```python
from build123d import *

# Parameters (mm, degrees)
SKETCH1_R                                  = 3
BOSS_EXTRUDE1_DEPTH                        = 275
SKETCH3_W                                  = 0.8
SKETCH3_H                                  = 0.5
CUT_EXTRUDE2_DEPTH                         = 276.032725326
CUT_EXTRUDE2_DEPTH_BACK                    = 276.032725326
SKETCH4_W                                  = 3.470061058
SKETCH4_H                                  = 7
SKETCH4_W_2                                = 2.92528695
CHAMFER1_SIZE                              = 0.3
RETAINING_GROOVES_D5P7_1_START             = 7.05
SKETCH5_R                                  = 2.85
SKETCH5_R_2                                = 2.49
RETAINING_GROOVES_D5P7_1_DEPTH             = 0.8
RETAINING_GROOVES_D5P7_2_START             = 13
SKETCH6_R                                  = 2.85
SKETCH6_R_2                                = 2.49
RETAINING_GROOVES_D5P7_2_DEPTH             = 0.8
RETAINING_GROOVES_D5P7_3_START             = 260.25
SKETCH7_R                                  = 2.85
SKETCH7_R_2                                = 2.49
RETAINING_GROOVES_D5P7_3_DEPTH             = 0.8
RETAINING_GROOVES_D5P7_4_START             = 266.2
SKETCH8_R                                  = 2.85
SKETCH8_R_2                                = 2.49
RETAINING_GROOVES_D5P7_4_DEPTH             = 0.8
TWO_HUB_CROSS_PIN_D2_DEPTH                 = 276.032725326
TWO_HUB_CROSS_PIN_D2_DEPTH_BACK            = 276.032725326
SKETCH9_R                                  = 1
SKETCH10_R                                 = 3.1
REVB_LOWER_SHAFT_NOSE_CLEARANCE_2MM_DEPTH  = 2
REVB_OLDHAM_D2_DRIVE_PIN_CLOCKED_HOLE_OU_W = 1
REVB_OLDHAM_D2_DRIVE_PIN_CLOCKED_HOLE_OU_H = 6.000106441


# Read off the part's stored shape, not the designer's step: RevB_Oldham_D2_Drive_Pin_Clocked_Hole
with BuildPart() as part:
    # Sketch1 → Boss-Extrude1 (new body)
    with BuildSketch(Plane.XY):
        Circle(SKETCH1_R)
    extrude(amount=BOSS_EXTRUDE1_DEPTH)

    # Sketch3 → Cut-Revolve1 (revolve, cut)
    with BuildSketch(Plane(origin=(0, 0, 0), x_dir=(0, 0, -1), z_dir=(1, 0, 0)), mode=Mode.PRIVATE) as cut_revolve1_sk:
        with Locations((-266.6, 2.75)):
            Rectangle(SKETCH3_W, SKETCH3_H)
        with Locations((-260.65, 2.75)):
            Rectangle(SKETCH3_W, SKETCH3_H)
        with Locations((-13.4, 2.75)):
            Rectangle(SKETCH3_W, SKETCH3_H)
        with Locations((-7.45, 2.75)):
            Rectangle(SKETCH3_W, SKETCH3_H)
    revolve(cut_revolve1_sk.sketch.rotate(Axis((0, 0, 263.365004794), (0, 0, -1)), 90), axis=Axis((0, 0, 263.365004794), (0, 0, -1)), mode=Mode.SUBTRACT)

    # Sketch4 → Cut-Extrude2 (cut, two sides: drawn at the far end of the back side and taken through both)
    with BuildSketch(Plane(origin=(0, 0, 0), x_dir=(1, 0, 0), z_dir=(0, 1, 0)).offset(-CUT_EXTRUDE2_DEPTH_BACK)):
        with Locations((4.235030529, -3.5)):
            Rectangle(SKETCH4_W, SKETCH4_H)
        with Locations((-3.962643475, -3.5)):
            Rectangle(SKETCH4_W_2, SKETCH4_H)
    extrude(amount=CUT_EXTRUDE2_DEPTH + CUT_EXTRUDE2_DEPTH_BACK, mode=Mode.SUBTRACT)

    # Chamfer1
    chamfer1_edges = [part.edges().sort_by_distance(p)[0] for p in [
        (0, 3, 0),
        (0, -3, 0),
    ]]
    chamfer(chamfer1_edges, length=CHAMFER1_SIZE)

    # Sketch5 → Retaining_Grooves_D5p7_1 (add)
    with BuildSketch(Plane.XY.offset(RETAINING_GROOVES_D5P7_1_START)):
        Circle(SKETCH5_R)
        Circle(SKETCH5_R_2, mode=Mode.SUBTRACT)
    extrude(amount=RETAINING_GROOVES_D5P7_1_DEPTH)

    # Sketch6 → Retaining_Grooves_D5p7_2 (add)
    with BuildSketch(Plane.XY.offset(RETAINING_GROOVES_D5P7_2_START)):
        Circle(SKETCH6_R)
        Circle(SKETCH6_R_2, mode=Mode.SUBTRACT)
    extrude(amount=RETAINING_GROOVES_D5P7_2_DEPTH)

    # Sketch7 → Retaining_Grooves_D5p7_3 (add)
    with BuildSketch(Plane.XY.offset(RETAINING_GROOVES_D5P7_3_START)):
        Circle(SKETCH7_R)
        Circle(SKETCH7_R_2, mode=Mode.SUBTRACT)
    extrude(amount=RETAINING_GROOVES_D5P7_3_DEPTH)

    # Sketch8 → Retaining_Grooves_D5p7_4 (add)
    with BuildSketch(Plane.XY.offset(RETAINING_GROOVES_D5P7_4_START)):
        Circle(SKETCH8_R)
        Circle(SKETCH8_R_2, mode=Mode.SUBTRACT)
    extrude(amount=RETAINING_GROOVES_D5P7_4_DEPTH)

    # Sketch9 → Two_Hub_Cross_Pin_D2 (cut, two sides: drawn at the far end of the back side and taken through both)
    with BuildSketch(Plane(origin=(0, 0, 0), x_dir=(0, 0, -1), z_dir=(1, 0, 0)).offset(-TWO_HUB_CROSS_PIN_D2_DEPTH_BACK)):
        with Locations((-41.5, 0)):
            Circle(SKETCH9_R)
        with Locations((-243.5, 0)):
            Circle(SKETCH9_R)
    extrude(amount=TWO_HUB_CROSS_PIN_D2_DEPTH + TWO_HUB_CROSS_PIN_D2_DEPTH_BACK, mode=Mode.SUBTRACT)

    # Sketch10 → RevB_Lower_Shaft_Nose_Clearance_2mm (cut)
    with BuildSketch(Plane(origin=(0, 0, 0), x_dir=(-1, 0, 0), z_dir=(0, 0, -1))):
        Circle(SKETCH10_R)
    extrude(amount=-REVB_LOWER_SHAFT_NOSE_CLEARANCE_2MM_DEPTH, mode=Mode.SUBTRACT)

    # RevB_Oldham_D2_Drive_Pin_Clocked_Hole ou → RevB_Oldham_D2_Drive_Pin_Clocked_Hole (revolve, cut)
    with BuildSketch(Plane(origin=(0, 0, 22.925), x_dir=(0.2727065426398811, 0.962097262027807, 0), z_dir=(0, 0, -1))):
        with Locations((0.5, 2.6843e-05)):
            Rectangle(REVB_OLDHAM_D2_DRIVE_PIN_CLOCKED_HOLE_OU_W, REVB_OLDHAM_D2_DRIVE_PIN_CLOCKED_HOLE_OU_H)
    revolve(axis=Axis((0, 0, 22.925), (0.962097262027807, -0.2727065426398811, 0)), mode=Mode.SUBTRACT)


solid = part.part
```
Model file for the job. Use its own axes, mm. Give positions to 0.01 mm unless a question says otherwise; leave off trailing zeros. Order: outer loops, then holes, each group sorted by start corner. A loop starts at its lowest first (then second) coordinate and runs counter-clockwise, first axis right, second up.
1) Saw through at A-A, the plane z = 115. Write the cut outline in (x, y), then the cut area to 3 significant figures.
2) Pin check, flat tips, straight feed: pin 1 (1 mm diameter, centred on x = -2, z = 167.5, fed in from +Y); pin 2 (3.5 mm diameter, centred on y = -0.5, z = 4, fed in from -X); pin 3 (1.7 mm diameter, centred on y = -0.5, z = 5.5, fed in from +X). Stop position of each tip, or through.
3) Wall check: probe 1 along Z at (x, y) = (0.5, 0); probe 2 along Z at (x, y) = (1.5, 2.5); probe 3 along Y at (x, z) = (-0.75, 41.5). Give the ranges that are in metal, low to high.
4) Saw through at B-B, the plane x = -1.5. Count the separate pieces of the cut face and the enclosed holes in it, then the cut area to 3 significant figures.
Computed:
1. outline: circle Ø6 at (0, 0)
1. area: 28.3 mm2
2. pin 1: stops at y = 2.6
2. pin 2: stops at x = -2.5
2. pin 3: stops at x = 2.5
3. probe 1: z = 2 to 21.93, 23.92 to 40.5, 42.5 to 242.5, 244.5 to 275
3. probe 2: z = 2 to 7.05, 7.85 to 13, 13.8 to 260.25, 261.05 to 266.2, 267 to 275
3. probe 3: y = -2.9 to -1, 1 to 2.9
4. separate pieces: 1
4. enclosed holes: 3
4. area: 1,410 mm2
